The model under review builds one solid part; all positions refer to its coordinate system, in mm. A direction names the side the tool comes from. Round coordinates to 2 decimals unless told otherwise and drop trailing zeros. Write each loop counter-clockwise with the first axis right and the second up, starting at its lowest first coordinate (ties: lowest second). Pieces come first, ordered by that corner, then holes. Notation, with made-up numbers: M 88.5,26.5 L 125.5,26.5 A20 cw 125.5,56.5 Z; hole C 3.5,-2 d10. An arc over 180 degrees is marked long. Write item = value, one per line. Start each with the question number.
Item 1: For pin 1 Ø4.5 at (x, z) = (-10, 44.5) entering from +Y; pin 2 Ø6 at (x, z) = (43.5, 46.5) entering from -Y; pin 3 Ø12.5 at (x, y) = (-16.5, 33.5) entering from +Z; pin 4 Ø20 at (x, z) = (-37.5, 58) entering from +Y, all flat-tipped, find the tip position at first contact; note any pin that passes through.
Item 2: The part is to be moulded in two halves that separate along X. For faces 4 (the flat face through (-1, 0, 46)), 5 (the flat face through (76, -76.2, 38)), 6 (the flat face through (-88.9, -4, 38)), say which applies: +X half, -X half, draft (parallel to the pull), parting line (faces both ways), or undercut.
Item 3: To check wall thickness, follow line 1 along X through (y, z) = (39, 43); line 2 along Y through (x, z) = (72, 48); line 3 along X through (y, z) = (2.75, 38.1). State the ranges of each line that lie inside material, in increasing order.
Item 4: Take a section at D-D, the plane z = 19.5. Give the boundary of the cut face in (x, y), plus the area to 3 significant figures.
Item 5: Tool access review of faces 1 (the flat face through (-70, 60.25, 38)), 2 (the flat face through (-59, 41.2, 41)), 3 (the flat face through (-63.5, 63, 38)): name each direction out of +Z, -Z, +X, -X, +Y, -Y from which nothing blocks a thin tool from reaching the whole face with its end or side.
Item 6: Take a section at C-C, the plane y = -63.5. Give the boundary of the cut face in (x, z).
Item 7: Take a section at B-B, the plane x = -72. Give the boundary of the cut face in (y, z), plus the area to 3 significant figures.
from build123d import *

# Parameters (mm, degrees)
BOSS_EXTRUDE1_DEPTH = 76.2
SKETCH2_W           = 6.35
SKETCH2_H           = 41.2
BOSS_EXTRUDE2_DEPTH = 127
SKETCH3_R           = 6.35
CUT_EXTRUDE1_DEPTH  = 105.2


with BuildPart() as part:
    # Sketch1 → Boss-Extrude1 (new body)
    with BuildSketch(Plane.XY):
        Polygon((-63.5, 0), (63.5, 0), (63.5, -76.2), (88.9, -76.2), (88.9, 66.6), (63.5, 66.6), (63.5, 60.25), (76.2, 60.25), (76.2, 53.9), (63.5, 53.9), (63.5, 12.7), (-6.371461067, 12.7), (-6.371461067, 41.2), (-15.5, 41.2), (-15.5, 12.7), (-55.5, 12.7), (-55.5, 41.2), (-63.5, 41.2), (-63.5, 53.9), (-76.2, 53.9), (-76.2, 60.25), (-63.5, 60.25), (-63.5, 66.6), (-88.9, 66.6), (-88.9, -76.2), (-63.5, -76.2), align=None)
    extrude(amount=BOSS_EXTRUDE1_DEPTH)

    # Sketch2 → Boss-Extrude2 (add)
    with BuildSketch(Plane.ZY.offset(-63.5)):
        with Locations((3.175, 33.3)):
            Rectangle(SKETCH2_W, SKETCH2_H)
    extrude(amount=BOSS_EXTRUDE2_DEPTH)

    # Sketch3 → Cut-Extrude1 (cut)
    with BuildSketch(Plane.XZ):
        with Locations(Location((0, 38.1, 0), (0, 0, 270))):
            Circle(SKETCH3_R)
    extrude(amount=-CUT_EXTRUDE1_DEPTH, mode=Mode.SUBTRACT)


solid = part.part
Response values:
q1.pin_1 = 41.2
q1.pin_2 = 0
q1.pin_3 = 76.2
q1.pin_4 = 12.7
q2.face_4 = undercut
q2.face_5 = draft
q2.face_6 = -X half
q3.line_1 = -88.9 to -55.5, -15.5 to -6.37, 63.5 to 88.9
q3.line_2 = -76.2 to 53.9, 60.25 to 66.6
q3.line_3 = -88.9 to -6.35, 6.35 to 88.9
q4.outline = M -88.9,-76.2 L -63.5,-76.2 L -63.5,0 L 63.5,0 L 63.5,-76.2 L 88.9,-76.2 L 88.9,66.6 L 63.5,66.6 L 63.5,60.25 L 76.2,60.25 L 76.2,53.9 L 63.5,53.9 L 63.5,12.7 L -6.37,12.7 L -6.37,41.2 L -15.5,41.2 L -15.5,12.7 L -55.5,12.7 L -55.5,41.2 L -63.5,41.2 L -63.5,53.9 L -76.2,53.9 L -76.2,60.25 L -63.5,60.25 L -63.5,66.6 L -88.9,66.6 Z
q4.area = 9,190 mm2
q5.face_1 = +Z, -Z
q5.face_2 = +Z, +Y
q5.face_3 = +Z, -Z, +Y
q6.outline = M -88.9,0 L -63.5,0 L -63.5,76.2 L -88.9,76.2 Z; M 63.5,0 L 88.9,0 L 88.9,76.2 L 63.5,76.2 Z
q7.outline = M -76.2,0 L 53.9,0 L 53.9,76.2 L -76.2,76.2 Z; M 60.25,0 L 66.6,0 L 66.6,76.2 L 60.25,76.2 Z
q7.area = 10,400 mm2
